The listing builds one solid part. Answer for the finished solid, in the listing's coordinates (mm). A direction names the side the tool comes from. Give positions to 0.01 mm unless a question says otherwise; leave off trailing zeros. Write each loop counter-clockwise with the first axis right and the second up, starting at its lowest first coordinate (ties: lowest second). Pieces come first, ordered by that corner, then holes. Notation, with made-up numbers: (35, 43) - (52, 43) arc R14 cw to (52, 70) - close; hole circle Ø11 at (10, 19). An arc over 180 degrees is marked (long way). Answer in a Markdown table with one row per item. Add a question column.
from build123d import *

# Parameters (mm, degrees)
SKETCH1_W           = 36.957
SKETCH1_H           = 21.3995
SKETCH1_R           = 1.190625
SKETCH1_R_2         = 0.9525
BOSS_EXTRUDE1_DEPTH = 2.38125
BOSS_EXTRUDE3_DEPTH = 2.38125
CUT_EXTRUDE2_REACH  = 4.381
SKETCH4_R           = 2.4892
FILLET1_R           = 2.54


with BuildPart() as part:
    # Sketch1 → Boss-Extrude1 (new body)
    with BuildSketch(Plane.XY):
        with Locations((16.891, 9.11225)):
            Rectangle(SKETCH1_W, SKETCH1_H)
        with Locations((1.5875, 14.25575)):
            Circle(SKETCH1_R, mode=Mode.SUBTRACT)
        with Locations((32.1945, 1.5875)):
            Circle(SKETCH1_R_2, mode=Mode.SUBTRACT)
    extrude(amount=BOSS_EXTRUDE1_DEPTH)

    # Sketch2 → Boss-Extrude3 (add)
    with BuildSketch(Plane.XZ.offset(1.5875)):
        Polygon((-1.5875, 2.38125), (35.3695, 2.38125), (35.3695, 0), (20.409545256, 0), (2.210283942, -31.522045256), (-14.2875, -21.997045256), (-1.5875, 0), align=None)
    extrude(amount=BOSS_EXTRUDE3_DEPTH)

    # Sketch4 → Cut-Extrude2 (cut, up to next)
    with BuildSketch(Plane(origin=(0, -1.5875, 0), x_dir=(1, 0, 0), z_dir=(0, 1, 0)), mode=Mode.PRIVATE) as cut_extrude2_sk1:
        with Locations((-2.018977372, 19.797340731)):
            Circle(SKETCH4_R)
    cut_extrude2_tool1 = extrude(cut_extrude2_sk1.sketch, amount=-CUT_EXTRUDE2_REACH, mode=Mode.PRIVATE) & part.part
    add(cut_extrude2_tool1.solids().sort_by_distance((-2.018977, -1.5875, -19.797341))[0], mode=Mode.SUBTRACT)
    # Sketch4 → Cut-Extrude2 (cut, up to next)
    with BuildSketch(Plane(origin=(0, -1.5875, 0), x_dir=(1, 0, 0), z_dir=(0, 1, 0)), mode=Mode.PRIVATE) as cut_extrude2_sk2:
        with Locations((4.331022628, 8.798818102)):
            Circle(SKETCH4_R)
    cut_extrude2_tool2 = extrude(cut_extrude2_sk2.sketch, amount=-CUT_EXTRUDE2_REACH, mode=Mode.PRIVATE) & part.part
    add(cut_extrude2_tool2.solids().sort_by_distance((4.331023, -1.5875, -8.798818))[0], mode=Mode.SUBTRACT)

    # Fillet1
    fillet1_edges = [part.edges().sort_by_distance(p)[0] for p in [
        (9.411022628, -1.5875, 0),
    ]]
    fillet(fillet1_edges, radius=FILLET1_R)


solid = part.part
1. Section D-D (x = 22) is taken. Give the vertices of the cut face in (y, z).
2. Section A-A (x = -2.5) is taken. Give the vertices of the cut face in (y, z).
3. The mould has two halves that part along Z. Classify faces 1 (the face through (35.37, 8, 1)), 2 (the face through (0.355, -2.761, -20.545)), 3 (the face through (-8.026, -2.567, -11.153)): +Z half, -Z half, draft (parallel to the pull), parting line (faces both ways), or undercut.
4. Given pin 1 Ø1.7 at (x, y) = (32.19, 1.59) entering from -Z (1 decimal); pin 2 Ø1 at (x, y) = (19, 1.5) entering from -Z; pin 3 Ø1.2 at (y, z) = (10, 1) entering from -X; pin 4 Ø8 at (x, z) = (4.33, -8.8) entering from +Y, each flat-ended and moving along its own axis, determine where each tip first touches the part or whether it passes through.
5. Straight lines are drawn through the part: L1, parallel to Z at x = 17, y = 16.75; L2, parallel to X at y = 17.5, z = 1; L3, parallel to Y at x = 8, z = -7.5. For each, find the intervals that lie inside material, in ascending order. Write a range as [from, to].
6. Section C-C (x = 15) is taken. Give the vertices of the cut face in (y, z).
7. A tool of negligible diameter and unlimited length cuts with its end or side. For faces 4 (the face through (-1.588, 8, 1)), 5 (the face through (-5.92, -2.76, -26.83)), 6 (the face through (3, -1.588, -14)), from which of +Z, -Z, +X, -X, +Y, -Y can it reach the whole face along a straight path? Write none if from no direction.
8. Section B-B (y = 3.5) is taken. Give the vertices of the cut face in (x, z).
Geometry check:
| question | item | result |
|---|---|---|
| 1 | outline | (-3.97, 0) - (19.81, 0) - (19.81, 2.38) - (-3.97, 2.38) - close |
| 2 | outline | (-3.97, -28.8) - (-1.59, -28.8) - (-1.59, -22.24) - (-3.97, -22.24) - close; (-3.97, -17.36) - (-1.59, -17.36) - (-1.59, -2.54) arc R2.54 cw to (-1.4, -1.58) - (-3.97, -1.58) - close |
| 3 | face 1 | draft |
| 3 | face 2 | undercut |
| 3 | face 3 | +Z half |
| 4 | pin 1 | through |
| 4 | pin 2 | z = 0 |
| 4 | pin 3 | x = -1.59 |
| 4 | pin 4 | y = -1.59 |
| 5 | L1 | [0, 2.38] |
| 5 | L2 | [-1.59, 35.37] |
| 5 | L3 | [-3.97, -1.59] |
| 6 | outline | (-3.97, -9.37) - (-1.59, -9.37) - (-1.59, -2.54) arc R2.54 cw to (0.95, 0) - (19.81, 0) - (19.81, 2.38) - (-3.97, 2.38) - close |
| 7 | face 4 | +Z, -X, +Y, -Y |
| 7 | face 5 | -Z, -X, +Y, -Y |
| 7 | face 6 | -Z, +X, -X, +Y |
| 8 | outline | (-1.59, 0) - (35.37, 0) - (35.37, 2.38) - (-1.59, 2.38) - close |
